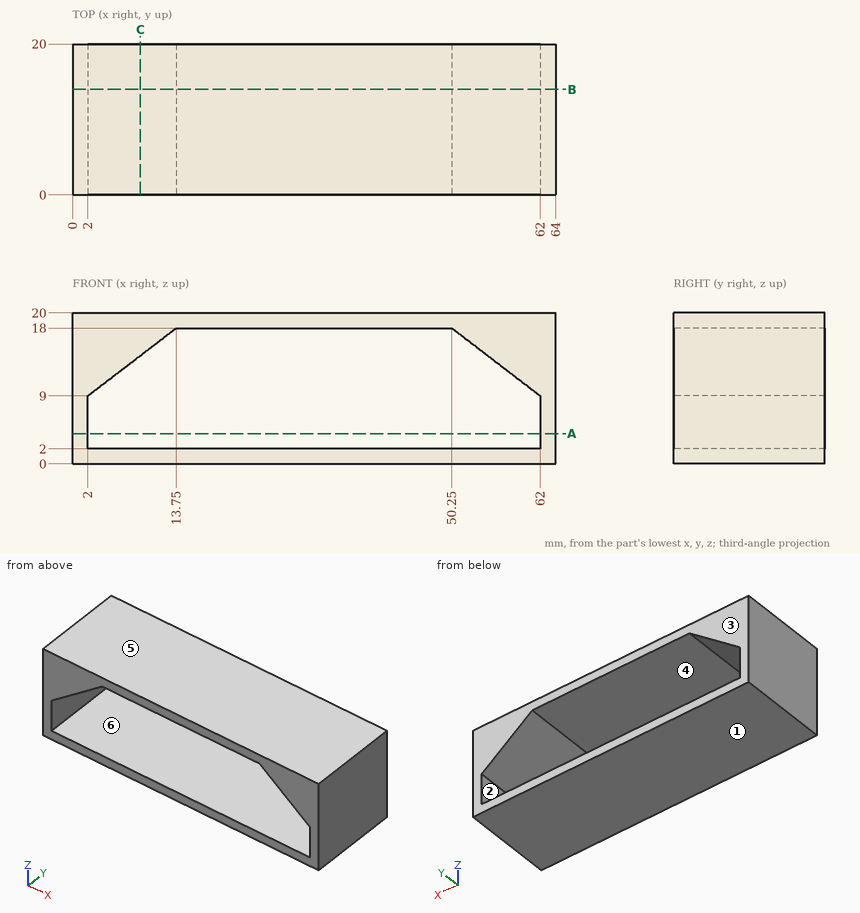
Print and shaded views of the part. All mm, measured from the part's lowest x, y and z. A direction names the side the tool comes from. Give positions to 0.01 mm unless a question says otherwise; leave off trailing zeros. Order: outer loops, then holes, each group sorted by start corner. A loop starts at its lowest first (then second) coordinate and runs counter-clockwise, first axis right, second up. Notation, with made-up numbers: (12, 68) -> (40, 68) arc R13 ccw to (40, 73) -> close; hole circle Ø10 at (16, 43.5). An arc over 180 degrees is marked (long way). Use CSV: the item, a comma, the result in double quotes.
1. Band-saw the part on A-A, the plane z = 4. Give the cut face in (x, y), then the cut area to 3 significant figures.
Outcome:
outline,"(0, 0) -> (2, 0) -> (2, 20) -> (0, 20) -> close; (62, 0) -> (64, 0) -> (64, 20) -> (62, 20) -> close"
area,"80.0 mm²"
2. Band-saw the part on B-B, the plane y = 14. Give the cut face in (x, z), then the cut area to 3 significant figures.
Outcome:
outline,"(0, 0) -> (64, 0) -> (64, 20) -> (0, 20) -> close; hole (2, 2) -> (62, 2) -> (62, 9) -> (50.25, 18) -> (13.75, 18) -> (2, 9) -> close"
area,"426 mm²"
3. Mould opens along Z. For the marked faces 1, 2, 3 and 4 say: +Z half, -Z half, draft (parallel to the pull), parting line (faces both ways), or undercut.
Outcome:
face 1,"-Z half"
face 2,"undercut"
face 3,"draft"
face 4,"undercut"
4. 3-axis set-ups, long thin cutter, end or side, ignore diameter. For the marked faces 5 and 6: which of +Z, -Z, +X, -X, +Y, -Y reach the whole face in a straight line?
Outcome:
face 5,"+Z, +X, -X, +Y, -Y"
face 6,"+Y, -Y"
5. Band-saw the part on C-C, the plane x = 9. Give the cut face in (y, z).
Outcome:
outline,"(0, 0) -> (20, 0) -> (20, 2) -> (0, 2) -> close; (0, 14.36) -> (20, 14.36) -> (20, 20) -> (0, 20) -> close"
6. Drill centre lines: line 1 along X through (y, z) = (2, 4.25); line 2 along Z through (x, y) = (18, 16.75); line 3 along X through (y, z) = (2.75, 11.25). Where is each one in solid material? Low to high. Write a range as from..to.
Outcome:
line 1,"0..2, 62..64"
line 2,"0..2, 18..20"
line 3,"0..4.94, 59.06..64"
